Input: part model. Units: mm. Frame: model coordinates. Coordinates: 2 decimals unless noted, no trailing zeros. Write each loop counter-clockwise with the first axis right and the second up, starting at its lowest first coordinate (ties: lowest second). Pieces come first, ordered by that corner, then holes. Notation, with made-up numbers: (6.25, -22.75) -> (57.25, -22.75) arc R16 cw to (57.25, -10.75) -> close; hole circle Ø1 at (-0.5, -20). An arc over 180 degrees is marked (long way). Use one line per item in the form item = value. Start each with the question number.
(1) Cut plane D-D on z = 36. Return the cut outline in (x, y).
(2) Cut plane B-B on y = -16.75. Return the cut outline in (x, z), plus the area to 3 significant figures.
(3) Pull-direction query (X, two-part tool) for faces 1 (the face through (56.577, -9.392, -11.582)), 2 (the face through (37.7, -9.4, 4)), 3 (the face through (41, 0, -1)); classes: released by +X, released by -X, zero draft, split by the parting line, or undercut.
(4) First-contact query: pin 1 (5 mm diameter, centred on y = -5.5, z = 24, fed in from -X); pin 2 (2 mm diameter, centred on y = -12.5, z = -20.5, fed in from -X); pin 3 (1.5 mm diameter, centred on y = -15.5, z = 32.5, fed in from -X). Flat tips, straight axial feed; report the tip coordinate or a pass-through.
(5) Ray query, line 1 along Z through (x, y) = (39, -8.25); line 2 along Z through (x, y) = (27, -1.5); line 3 along X through (y, z) = (-2, -6.5). Return the intervals inside material, ascending.
(6) Cut plane A-A on x = 43. Return the cut outline in (y, z), plus the area to 3 significant figures.
(7) Cut plane C-C on z = 4. Return the cut outline in (x, y), plus the area to 3 significant figures.
```python
from build123d import *

# Parameters (mm, degrees)
F1_DEPTH = 19.05


with BuildPart() as f1:
    # F0 (on Front) → F1 (new body)
    with BuildSketch(Plane.XZ):
        with BuildLine():
            ThreePointArc((36.753029, 40.957993), (37.281433, 3.593556), (0, 6.138184))
            ThreePointArc((0, 6.138184), (8.90252, -6.437058), (23.138397, -12.330394))
            ThreePointArc((23.138397, -12.330394), (24.611231, -12.401927), (26.082398, -12.502042))
            ThreePointArc((26.082398, -12.502042), (43.391463, -6.559586), (53.243299, 8.863053))
            ThreePointArc((53.243299, 8.863053), (53.500008, 12.310691), (53.987336, 15.733354))
            ThreePointArc((53.987336, 15.733354), (49.151042, 30.928882), (36.753029, 40.957993))
        make_face()
        with BuildLine():
            ThreePointArc((26.082398, -12.502042), (24.611231, -12.401927), (23.138397, -12.330394))
            ThreePointArc((23.138397, -12.330394), (24.608117, -12.455329), (26.082398, -12.502042))
        make_face()
        with BuildLine():
            ThreePointArc((53.243299, 8.863053), (53.829881, 12.274967), (53.987336, 15.733354))
            ThreePointArc((53.987336, 15.733354), (53.500008, 12.310691), (53.243299, 8.863053))
        make_face()
        with BuildLine():
            ThreePointArc((53.243299, 8.863053), (43.391463, -6.559586), (26.082398, -12.502042))
            ThreePointArc((26.082398, -12.502042), (47.890891, -17.50496), (67.295052, -28.645788))
            ThreePointArc((67.295052, -28.645788), (56.475186, -11.312691), (53.243299, 8.863053))
        make_face()
    extrude(amount=F1_DEPTH)


solid = f1.part
```
Values:
q1.outline = (41.03, -19.05) -> (44.69, -19.05) -> (44.69, 0) -> (41.03, 0) -> close
q2.outline = (0, 6.14) arc R27.77 ccw to (23.14, -12.33) arc R27.77 ccw to (26.08, -12.5) arc R75.95 cw to (67.3, -28.65) arc R51.53 cw to (53.24, 8.86) arc R27.77 ccw to (53.99, 15.73) arc R27.77 ccw to (36.75, 40.96) arc R25.4 cw (long way) to start
q2.area = 1,020 mm2
q3.face_1 = released by +X
q3.face_2 = undercut
q3.face_3 = zero draft
q4.pin_1 = 44.82
q4.pin_2 = 52.52
q4.pin_3 = 42.6
q5.line_1 = -14.64 to 5.39, 38.68 to 39.92
q5.line_2 = -12.58 to -2.33
q5.line_3 = 8.98 to 54.94
q6.outline = (-19.05, -15.78) -> (0, -15.78) -> (0, 11.66) -> (-19.05, 11.66) -> close; (-19.05, 32.4) -> (0, 32.4) -> (0, 37.39) -> (-19.05, 37.39) -> close
q6.area = 618 mm2
q7.outline = (0.84, -19.05) -> (1.92, -19.05) -> (1.92, 0) -> (0.84, 0) -> close; (37.7, -19.05) -> (53.27, -19.05) -> (53.27, 0) -> (37.7, 0) -> close
q7.area = 317 mm2
